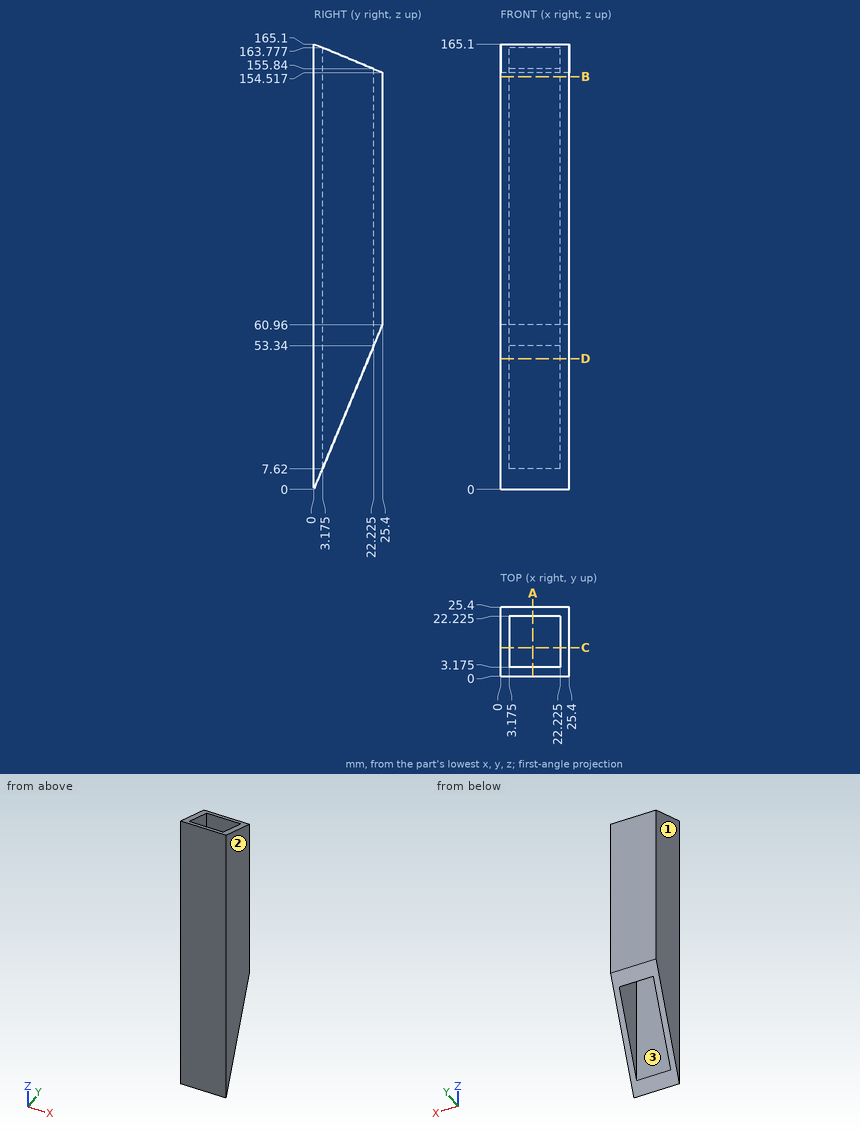
Design review of the part shown in the three views and the two pictorial views. Dimensions are in mm from the part's minimum x, y and z. Round coordinates to 2 decimals unless told otherwise and drop trailing zeros. Write each loop counter-clockwise with the first axis right and the second up, starting at its lowest first coordinate (ties: lowest second). Pieces come first, ordered by that corner, then holes. Notation, with made-up numbers: (78.25, 48.5) - (121.25, 48.5) arc R15 ccw to (121.25, 69.5) - close; hole circle Ø2 at (32.5, -17.5). An arc over 180 degrees is marked (long way). Answer as CSV lines item,"result". Start each with the question number.
(1) For pin 1 (1.5 mm diameter, centred on x = 4.5, y = 3, fed in from +Z); pin 2 (6 mm diameter, centred on x = 21, y = 9, fed in from +Z); pin 3 (10 mm diameter, centred on y = 20, z = 30, fed in from -X); pin 4 (3 mm diameter, centred on x = 3, y = 22.5, fed in from -Z), all flat-tipped, find the tip position at first contact; note any pin that passes through.
(2) Add section C-C, the plane y = 10.5. State the section outline as (x, z) points (1 decimal).
(3) Add section B-B, the plane z = 153. State the section outline as (x, y) points (1 decimal).
(4) For line 1 (X direction, y = 7, z = 98.5) (1 decimal); line 2 (Y direction, x = 6.75, z = 26.5) (1 decimal), list the stretches that pass through material, from the lowest coordinate up.
(5) Add section D-D, the plane z = 48.5. State the section outline as (x, y) points (1 decimal).
(6) Mouldability with a two-part tool opening along X and no side actions: class the marked faces 1, 2 and 3 as +X half, -X half, draft (parallel to the pull), parting line (faces both ways), or undercut.
(7) Add section A-A, the plane x = 12. State the section outline as (y, z) points (1 decimal).
From the geometry:
1,pin 1,"stops at z = 164.16"
1,pin 2,"stops at z = 162.49"
1,pin 3,"passes through"
1,pin 4,"stops at z = 50.4"
2,outline,"(0, 25.2) - (3.2, 25.2) - (3.2, 160.7) - (0, 160.7) - close; (22.2, 25.2) - (25.4, 25.2) - (25.4, 160.7) - (22.2, 160.7) - close"
3,outline,"(0, 0) - (25.4, 0) - (25.4, 25.4) - (0, 25.4) - close; hole (3.2, 3.2) - (22.2, 3.2) - (22.2, 22.2) - (3.2, 22.2) - close"
4,line 1,"x = 0 to 3.2, 22.2 to 25.4"
4,line 2,"y = 0 to 3.2"
5,outline,"(0, 0) - (25.4, 0) - (25.4, 20.2) - (22.2, 20.2) - (22.2, 3.2) - (3.2, 3.2) - (3.2, 20.2) - (0, 20.2) - close"
6,face 1,"-X half"
6,face 2,"+X half"
6,face 3,"undercut"
7,outline,"(0, 0) - (3.2, 7.6) - (3.2, 163.8) - (0, 165.1) - close; (22.2, 53.3) - (25.4, 61) - (25.4, 154.5) - (22.2, 155.8) - close"
